from build123d import *

# Parameters (mm, degrees)
SKETCH1_R           = 17.526
SKETCH1_R_2         = 3.96875
BOSS_EXTRUDE1_DEPTH = 6.35
CHAMFER2_SIZE       = 0.254
BOSS_EXTRUDE2_START = 6.35
SKETCH3_R           = 9.525
SKETCH3_R_2         = 3.96875
BOSS_EXTRUDE2_DEPTH = 6.35
CHAMFER3_SIZE       = 0.508
SKETCH8_R           = 12.7
SKETCH8_R_2         = 4.22275
BOSS_EXTRUDE3_DEPTH = 14.224
SKETCH6_R           = 1.9685
CUT_EXTRUDE2_DEPTH  = 16.764


with BuildPart() as part:
    # Sketch1 → Boss-Extrude1 (new body)
    with BuildSketch(Plane(origin=(0, 0, 0), x_dir=(0, 0, -1), z_dir=(1, 0, 0))):
        Circle(SKETCH1_R)
        Circle(SKETCH1_R_2, mode=Mode.SUBTRACT)
    extrude(amount=BOSS_EXTRUDE1_DEPTH)

    # Chamfer2
    chamfer2_edges = [part.edges().sort_by_distance(p)[0] for p in [
        (0, 0, 17.526),
        (6.35, 0, 17.526),
        (0, 0, 3.96875),
        (6.35, 0, 3.96875),
    ]]
    chamfer(chamfer2_edges, length=CHAMFER2_SIZE)

    # Sketch3 → Boss-Extrude2 (add)
    with BuildSketch(Plane.ZY.offset(BOSS_EXTRUDE2_START)):
        with Locations(Location((0, 0, 0), (0, 0, 180))):
            Circle(SKETCH3_R)
        with Locations(Location((0, 0, 0), (0, 0, 180))):
            Circle(SKETCH3_R_2, mode=Mode.SUBTRACT)
    extrude(amount=-BOSS_EXTRUDE2_DEPTH)

    # Chamfer3
    chamfer3_edges = [part.edges().sort_by_distance(p)[0] for p in [
        (0, 0, 9.525),
        (-6.35, 0, 9.525),
    ]]
    chamfer(chamfer3_edges, length=CHAMFER3_SIZE)

    # Sketch8 → Boss-Extrude3 (add)
    with BuildSketch(Plane(origin=(6.35, 0, 0), x_dir=(0, 0, -1), z_dir=(1, 0, 0))):
        Circle(SKETCH8_R)
        Circle(SKETCH8_R_2, mode=Mode.SUBTRACT)
    extrude(amount=BOSS_EXTRUDE3_DEPTH)

    # Sketch6 → Cut-Extrude2 (cut)
    with BuildSketch(Plane.XY):
        with Locations(Location((-3.175, 0, 0), (0, 0, 180))):
            Circle(SKETCH6_R)
        with Locations((13.462, 0)):
            Circle(SKETCH6_R)
    extrude(amount=-CUT_EXTRUDE2_DEPTH, mode=Mode.SUBTRACT)


solid = part.part
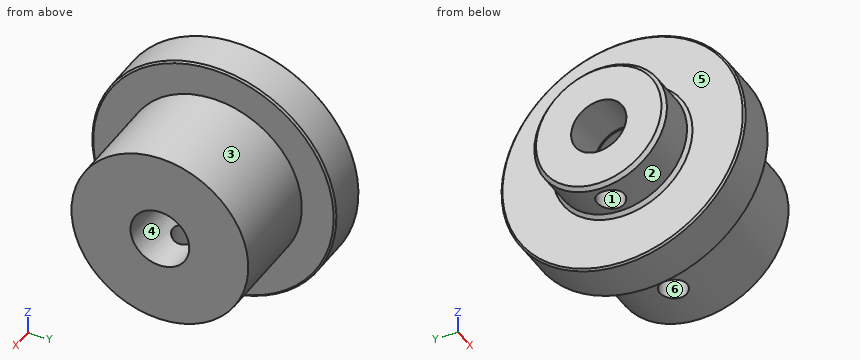
Source: CAD feature listing. Evaluate the final solid. Frame: model axes, mm. Face numbers are marked on the shaded views. A direction names the side the tool comes from. Coordinates: 2 decimals unless noted, no trailing zeros. Loops run counter-clockwise (first coordinate to the right, second up) from the corner with the lowest first, then second, coordinate; pieces in that order, holes last. Notation, with made-up numbers: M -15.75,54.25 L 8.25,54.25 A10 ccw 8.25,58.25 Z; hole C 42.25,-5.75 d4. An arc over 180 degrees is marked long. Answer in a Markdown table with one row per item.
Q1. Ray query, probe 1 along Y at (x, z) = (2.75, 0); probe 2 along Y at (x, z) = (13.25, 0); probe 3 along X at (y, z) = (13.5, -10). Return the intervals inside material, ascending. Write a range as from..to.
Answers below:
| item | result |
|---|---|
| probe 1 | y = -17.53..-3.97, 3.97..17.53 |
| probe 2 | y = -12.7..-4.22, 4.22..12.7 |
| probe 3 | x = 0..6.35 |
Q2. Section B-B on y = 0. State how many separate pieces and enclosed holes the cut face has, plus the area to 3 significant figures.
Answers below:
| item | result |
|---|---|
| separate pieces | 4 |
| enclosed holes | 0 |
| area | 428 mm^2 |
Q3. Set-up query: the marked faces 1, 2 and 3. Return all of +Z, -Z, +X, -X, +Y, -Y with unobstructed straight access to the full face (end or side cutting, diameter ignored); none if empty.
Answers below:
| item | result |
|---|---|
| face 1 | -Z |
| face 2 | -X |
| face 3 | +X |
Q4. First-contact query: pin 1 (8 mm diameter, centred on x = 10, y = -12, fed in from +Z); pin 2 (2.5 mm diameter, centred on x = -3.175, y = 0, fed in from -Z); pin 3 (2 mm diameter, centred on x = 5, y = -5, fed in from -Z). Flat tips, straight axial feed; report the tip coordinate or a pass-through.
Answers below:
| item | result |
|---|---|
| pin 1 | stops at z = 13.82 |
| pin 2 | stops at z = 3.77 |
| pin 3 | stops at z = -17.06 |
Q5. Section C-C on x = 3. Return the cut outline in (y, z).
Answers below:
| item | result |
|---|---|
| outline | C 0,0 d35.05; hole C 0,0 d7.94 |
Q6. Draft query along X for the marked faces 4, 5 and 6. Return one class per face: pulls with the +X half, pulls with the -X half, needs draft (parallel to the pull), parting line crosses it, or undercut.
Answers below:
| item | result |
|---|---|
| face 4 | needs draft |
| face 5 | pulls with the -X half |
| face 6 | undercut |
